```python
from build123d import *

# Parameters (mm, degrees)
SKETCH_1_W          = 101
SKETCH_1_H          = 74
SKETCH_1_R          = 1.5
EXTRUDE_1_DEPTH     = 2
SKETCH_2_W          = 58
SKETCH_2_H          = 26
CUT_EXTRUDE_1_DEPTH = 2
CUT_EXTRUDE_2_DEPTH = 2
EXTRUDE_2_DEPTH     = 2
CUT_EXTRUDE_3_DEPTH = 2
FILLET_1_R          = 2


with BuildPart() as part:
    # 草图1 → 凸台-拉伸1 (new body)
    with BuildSketch(Plane(origin=(0, 0, 0), x_dir=(1, 0, 0), z_dir=(0, 1, 0))):
        Rectangle(SKETCH_1_W, SKETCH_1_H)
        with Locations(Location((32, -16, 0), (0, 0, 270))):
            Circle(SKETCH_1_R, mode=Mode.SUBTRACT)
        with Locations(Location((32, 16, 0), (0, 0, 270))):
            Circle(SKETCH_1_R, mode=Mode.SUBTRACT)
        with Locations(Location((-32, 16, 0), (0, 0, 270))):
            Circle(SKETCH_1_R, mode=Mode.SUBTRACT)
        with Locations(Location((-32, -16, 0), (0, 0, 270))):
            Circle(SKETCH_1_R, mode=Mode.SUBTRACT)
        with Locations(Location((47.5, 34, 0), (0, 0, 270))):
            Circle(SKETCH_1_R, mode=Mode.SUBTRACT)
        with Locations(Location((-47.5, 34, 0), (0, 0, 270))):
            Circle(SKETCH_1_R, mode=Mode.SUBTRACT)
        with Locations(Location((-47.5, -34, 0), (0, 0, 270))):
            Circle(SKETCH_1_R, mode=Mode.SUBTRACT)
        with Locations(Location((47.5, -34, 0), (0, 0, 270))):
            Circle(SKETCH_1_R, mode=Mode.SUBTRACT)
    extrude(amount=EXTRUDE_1_DEPTH)

    # 草图2 → 切除-拉伸1 (cut)
    with BuildSketch(Plane(origin=(0, 2, 0), x_dir=(1, 0, 0), z_dir=(0, 1, 0))):
        Rectangle(SKETCH_2_W, SKETCH_2_H)
    extrude(amount=-CUT_EXTRUDE_1_DEPTH, mode=Mode.SUBTRACT)

    # 草图3 → 切除-拉伸2 (cut)
    with BuildSketch(Plane(origin=(0, 2, 0), x_dir=(1, 0, 0), z_dir=(0, 1, 0))):
        Polygon((-44.804678435, 37), (-28.443567324, 18), (28.443567324, 18), (44.804678435, 37), align=None)
    cut_extrude_2 = extrude(amount=-CUT_EXTRUDE_2_DEPTH, mode=Mode.SUBTRACT)

    # 镜向1: 切除-拉伸2 across plane
    add(cut_extrude_2.mirror(Plane.XY), mode=Mode.SUBTRACT)

    # 草图4 → 凸台-拉伸2 (add)
    with BuildSketch(Plane(origin=(0, 2, 0), x_dir=(1, 0, 0), z_dir=(0, 1, 0))):
        Polygon((0, -2.191758425), (-4.889307256, 0), (-29, -10.808241575), (-29, -13), (-24.110692744, -13), align=None)
        Polygon((-29, 13), (-29, 10.808241575), (-4.889307256, 0), (0, 2.191758425), (-24.110692744, 13), align=None)
        Polygon((0, 2.191758425), (-4.889307256, 0), (0, -2.191758425), (4.889307256, 0), align=None)
        Polygon((24.110692744, 13), (0, 2.191758425), (4.889307256, 0), (29, 10.808241575), (29, 13), align=None)
        Polygon((4.889307256, 0), (0, -2.191758425), (24.110692744, -13), (29, -13), (29, -10.808241575), align=None)
    extrude(amount=-EXTRUDE_2_DEPTH)

    # 草图5 → 切除-拉伸3 (cut)
    with BuildSketch(Plane.XZ):
        Polygon((-46.5, 28.241171541), (-35, 14.886332831), (-35, -14.886332831), (-46.5, -28.241171541), align=None)
    cut_extrude_3 = extrude(amount=-CUT_EXTRUDE_3_DEPTH, mode=Mode.SUBTRACT)

    # 镜向2: 切除-拉伸3 across plane
    add(cut_extrude_3.mirror(Plane(origin=(0, 0, 0), x_dir=(0, 0, 1), z_dir=(1, 0, 0))), mode=Mode.SUBTRACT)

    # 圆角1
    fillet_1_edges = [part.edges().sort_by_distance(p)[0] for p in [
        (0, 1, 2.191758425),
        (-24.110692744, 1, 13),
        (-29, 1, 10.808241575),
        (-4.889307256, 1, 0),
        (-29, 1, -10.808241575),
        (-24.110692744, 1, -13),
        (0, 1, -2.191758425),
        (24.110692744, 1, -13),
        (29, 1, -10.808241575),
        (4.889307256, 1, 0),
        (29, 1, 10.808241575),
        (24.110692744, 1, 13),
        (-46.5, 1, -28.241171541),
        (-46.5, 1, 28.241171541),
        (-35, 1, 14.886332831),
        (-35, 1, -14.886332831),
        (46.5, 1, 28.241171541),
        (46.5, 1, -28.241171541),
        (35, 1, -14.886332831),
        (35, 1, 14.886332831),
        (-44.804678435, 1, -37),
        (44.804678435, 1, -37),
        (28.443567324, 1, -18),
        (-28.443567324, 1, -18),
        (-50.5, 1, 37),
        (-50.5, 1, -37),
        (50.5, 1, -37),
        (50.5, 1, 37),
        (44.804678435, 1, 37),
        (-44.804678435, 1, 37),
        (-28.443567324, 1, 18),
        (28.443567324, 1, 18),
    ]]
    fillet(fillet_1_edges, radius=FILLET_1_R)


solid = part.part
```
Input: part model. Units: mm. Frame: model coordinates. A direction names the side the tool comes from. Give positions to 0.01 mm unless a question says otherwise; leave off trailing zeros. Write each loop counter-clockwise with the first axis right and the second up, starting at its lowest first coordinate (ties: lowest second). Pieces come first, ordered by that corner, then holes. Notation, with made-up numbers: (48.5, -6.5) - (100.5, -6.5) arc R14 ccw to (100.5, 20.5) - close; hole circle Ø11 at (37, 70.25). An arc over 180 degrees is marked (long way). Write item = value, one per line. Start each with the question number.
1. First-contact query: pin 1 Ø1 at (x, y) = (-18, 0.5) entering from +Z; pin 2 Ø2.5 at (x, z) = (-32, -16) entering from +Y; pin 3 Ø0.6 at (x, y) = (-5.5, 0.5) entering from -Z. Flat tips, straight axial feed; report the tip coordinate or a pass-through.
2. Access query for faces 4 (the flat face through (-35, 1, 0)), 5 (the flat face through (36.52, 1.01, 27.38)), 6 (the cylindrical face through (-49.93, 1.01, -36.4)). Directions: +Z, -Z, +X, -X, +Y, -Y. A direction counts if a zero-diameter tool reaches every point of the face in a straight line with its end or side. Return the directions, or none.
3. Section query C-C, the plane z = -4. Output: boundary loops of the cut face in (x, y), then the cut area to 3 significant figures.
4. Mould query, pull axis X, two halves, no side actions, for faces 1 (the cylindrical face through (49.9, 1.01, 36.43)), 2 (the flat face through (-36.73, 1.01, -27.62)), 3 (the flat face through (47, 1, -37)). Classes: released by +X, released by -X, zero draft, split by the parting line, or undercut.
5. Section query D-D, the plane x = 32. Output: boundary loops of the cut face in (y, z), then the cut area to 3 significant figures.
6. Ray query, L1, parallel to X at y = 1.8, z = 11; L2, parallel to Z at x = 31, y = 0.3; L3, parallel to X at y = 0.45, z = -6. Return the intervals inside material, ascending.
7. Section query A-A, the plane x = -24.5. Output: boundary loops of the cut face in (y, z), then the cut area to 3 significant figures.
8. Section query B-B, the plane y = 0.95. Count the separate pieces of the cut face and the enclosed holes in it, then the cut area to 3 significant figures.
Check sheet entries:
q1.pin_1 = 18
q1.pin_2 = through
q1.pin_3 = -18
q2.face_4 = +Y, -Y
q2.face_5 = +Z, +Y, -Y
q2.face_6 = -Z, -X, +Y, -Y
q3.outline = (-50.5, 0) - (-46.5, 0) - (-46.5, 2) - (-50.5, 2) - close; (-35, 0) - (-29, 0) - (-29, 2) - (-35, 2) - close; (-13.81, 0) - (-4.03, 0) - (-4.03, 2) - (-13.81, 2) - close; (4.03, 0) - (13.81, 0) - (13.81, 2) - (4.03, 2) - close; (29, 0) - (35, 0) - (35, 2) - (29, 2) - close; (46.5, 0) - (50.5, 0) - (50.5, 2) - (46.5, 2) - close
q3.area = 79.1 mm2
q4.face_1 = released by +X
q4.face_2 = undercut
q4.face_3 = zero draft
q5.outline = (0, -22.13) - (2, -22.13) - (2, -17.5) - (0, -17.5) - close; (0, -14.5) - (2, -14.5) - (2, 14.5) - (0, 14.5) - close; (0, 17.5) - (2, 17.5) - (2, 22.13) - (0, 22.13) - close
q5.area = 76.5 mm2
q6.L1 = -50.5 to -46.5, -35 to -16.76, 16.76 to 35, 46.5 to 50.5
q6.L2 = -20.97 to -17.12, -14.88 to 14.88, 17.12 to 20.97
q6.L3 = -50.5 to -46.5, -35 to -29, -18.27 to -8.5, 8.5 to 18.27, 29 to 35, 46.5 to 50.5
q7.outline = (0, -18) - (2, -18) - (2, -8.79) - (0, -8.79) - close; (0, 8.79) - (2, 8.79) - (2, 18) - (0, 18) - close
q7.area = 36.8 mm2
q8.separate_pieces = 1
q8.enclosed_holes = 14
q8.area = 2,690 mm2
